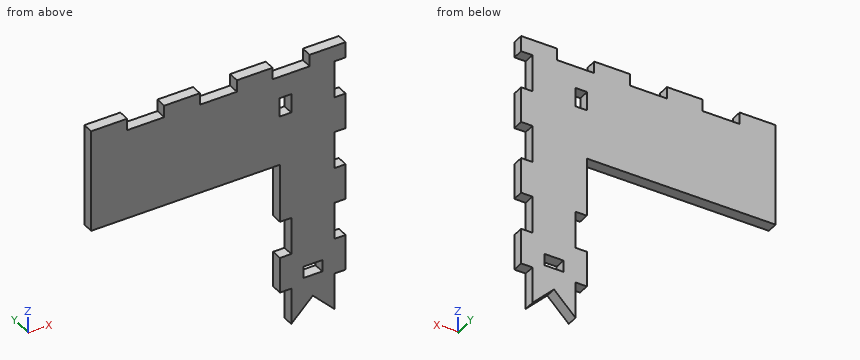
```python
from build123d import *

# Parameters (mm, degrees)
BOSS_EXTRUDE1_DEPTH = 3
SKETCH8_W           = 3.2
SKETCH8_H           = 10.2
SKETCH8_W_2         = 5.2
SKETCH8_H_2         = 3.2
SKETCH8_H_3         = 5.2
CUT_EXTRUDE4_DEPTH  = 4
CUT_EXTRUDE2_DEPTH  = 4


with BuildPart() as part:
    # Sketch1 → Boss-Extrude1 (new body)
    with BuildSketch(Plane(origin=(0, 0, 0), x_dir=(1, 0, 0), z_dir=(0, 1, 0))):
        Polygon((-34.872217102, 0), (34.872217102, 0), (34.872217102, 75), (16.872217102, 75), (16.872217102, 28.75), (-34.872217102, 28.75), align=None)
    extrude(amount=-BOSS_EXTRUDE1_DEPTH)

    # Sketch8 → Cut-Extrude4 (cut, through all)
    with BuildSketch(Plane(origin=(0, 0, 0), x_dir=(1, 0, 0), z_dir=(0, 1, 0))):
        with Locations((33.372217102, 50)):
            Rectangle(SKETCH8_W, SKETCH8_H)
        with Locations((33.372217102, 70)):
            Rectangle(SKETCH8_W, SKETCH8_H)
        with Locations((25.872217102, 61.5)):
            Rectangle(SKETCH8_W_2, SKETCH8_H_2)
        with Locations((33.372217102, 10)):
            Rectangle(SKETCH8_W, SKETCH8_H)
        with Locations((33.372217102, 30)):
            Rectangle(SKETCH8_W, SKETCH8_H)
        with Locations((18.372217102, 12.5)):
            Rectangle(SKETCH8_W, SKETCH8_H_3)
        with Locations((18.372217102, 70)):
            Rectangle(SKETCH8_W, SKETCH8_H)
        Polygon((-34.972217102, 0.6), (-34.972217102, -0.1), (34.972217102, -0.1), (34.972217102, 0.6), (25.008726501, 0.6), (25.008726501, 3.85), (14.845235901, 3.85), (14.845235901, 0.6), (5.0817453, 0.6), (5.0817453, 3.85), (-5.0817453, 3.85), (-5.0817453, 0.6), (-14.845235901, 0.6), (-14.845235901, 3.85), (-25.008726501, 3.85), (-25.008726501, 0.6), align=None)
        with Locations((18.372217102, 50)):
            Rectangle(SKETCH8_W, SKETCH8_H)
    extrude(amount=-CUT_EXTRUDE4_DEPTH, mode=Mode.SUBTRACT)

    # Sketch5 → Cut-Extrude2 (cut, through all)
    with BuildSketch(Plane(origin=(0, 0, 0), x_dir=(1, 0, 0), z_dir=(0, 1, 0))):
        Polygon((31.872217102, 75), (25.872217102, 69), (19.872217102, 75), align=None)
    extrude(amount=-CUT_EXTRUDE2_DEPTH, mode=Mode.SUBTRACT)


solid = part.part
```
Can you work these out from the model? Positions are in its coordinate system, mm. Coordinates: 2 decimals unless noted, no trailing zeros. Loops run counter-clockwise (first coordinate to the right, second up) from the corner with the lowest first, then second, coordinate; pieces in that order, holes last.
1) Imagine slicing it at D-D on x = -28.5. List the corners of the cut face in (y, z) for me.
2) Imagine slicing it at C-C on y = -0.9. State how many separate pieces and enclosed holes the cut face has, plus the area to 3 significant figures.
3) For pin 1 (1.5 mm diameter, centred on y = -2, z = -30, fed in from +X); pin 2 (1.5 mm diameter, centred on x = -20.5, y = -1, fed in from +Z); pin 3 (0.9 mm diameter, centred on x = 33.5, y = -1.5, fed in from -Z), each with a flat end and sliding along its axis, tell me the tip position at first contact or that it passes through.
4) Imagine slicing it at A-A on z = -12. List the corners of the cut face in (x, y) for me, plus the area to 3 significant figures.
5) Imagine slicing it at B-B on x = 19. List the corners of the cut face in (y, z) for me.
6) I need wall thicknesses on probe 1 along X at (y, z) = (-1.05, -30.5); probe 2 along Z at (x, y) = (6.5, -1.2); probe 3 along Z at (x, y) = (1, -0.9). Which ranges of each line are inside material? Lowest first, please.
Completed:
1. outline: (-3, -28.75) - (0, -28.75) - (0, -0.6) - (-3, -0.6) - close
2. separate pieces: 1
2. enclosed holes: 2
2. area: 2,440 mm2
3. pin 1: stops at x = 31.77
3. pin 2: stops at z = -3.85
3. pin 3: stops at z = -64.9
4. outline: (-34.87, -3) - (16.77, -3) - (16.77, 0) - (-34.87, 0) - close; (19.97, -3) - (31.77, -3) - (31.77, 0) - (19.97, 0) - close
4. area: 190 mm2
5. outline: (-3, -64.9) - (0, -64.9) - (0, -55.1) - (-3, -55.1) - close; (-3, -44.9) - (0, -44.9) - (0, -15.1) - (-3, -15.1) - close; (-3, -9.9) - (0, -9.9) - (0, -3.85) - (-3, -3.85) - close
6. probe 1: x = 16.87 to 31.77
6. probe 2: z = -28.75 to -0.6
6. probe 3: z = -28.75 to -3.85
